from build123d import *

# Parameters (mm, degrees)
SKETCH2_W           = 75
SKETCH2_H           = 60
BOSS_EXTRUDE1_DEPTH = 2
SKETCH4_R           = 1.5
SKETCH4_R_2         = 2
CUT_EXTRUDE2_DEPTH  = 2
SKETCH5_R           = 5
CUT_EXTRUDE3_DEPTH  = 40
FILLET1_R           = 1


with BuildPart() as part:
    # Sketch2 → Boss-Extrude1 (new body)
    with BuildSketch(Plane(origin=(0, 0, 0), x_dir=(1, 0, 0), z_dir=(0, 1, 0))):
        with Locations((37.5, 30)):
            Rectangle(SKETCH2_W, SKETCH2_H)
    extrude(amount=BOSS_EXTRUDE1_DEPTH)

    # Sketch4 → Cut-Extrude2 (cut)
    with BuildSketch(Plane(origin=(0, 2, 0), x_dir=(1, 0, 0), z_dir=(0, 1, 0))):
        with Locations(Location((10, 10, 0), (0, 0, 270))):
            Circle(SKETCH4_R)
        with Locations(Location((65, 10, 0), (0, 0, 270))):
            Circle(SKETCH4_R)
        with Locations(Location((20, 20, 0), (0, 0, 270))):
            Circle(SKETCH4_R_2)
        with Locations(Location((55, 20, 0), (0, 0, 270))):
            Circle(SKETCH4_R_2)
        with Locations(Location((10, 50, 0), (0, 0, 270))):
            Circle(SKETCH4_R)
        with Locations(Location((65, 50, 0), (0, 0, 270))):
            Circle(SKETCH4_R)
    extrude(amount=-CUT_EXTRUDE2_DEPTH, mode=Mode.SUBTRACT)

    # Sketch5 → Cut-Extrude3 (cut)
    with BuildSketch(Plane(origin=(0, 2, 0), x_dir=(1, 0, 0), z_dir=(0, 1, 0))):
        with Locations(Location((37.5, 28, 0), (0, 0, 270))):
            Circle(SKETCH5_R)
    extrude(amount=-CUT_EXTRUDE3_DEPTH, mode=Mode.SUBTRACT)

    # Fillet1
    fillet1_edges = [part.edges().sort_by_distance(p)[0] for p in [
        (0, 1, -60),
        (75, 1, -60),
        (75, 1, 0),
        (0, 1, 0),
    ]]
    fillet(fillet1_edges, radius=FILLET1_R)


solid = part.part
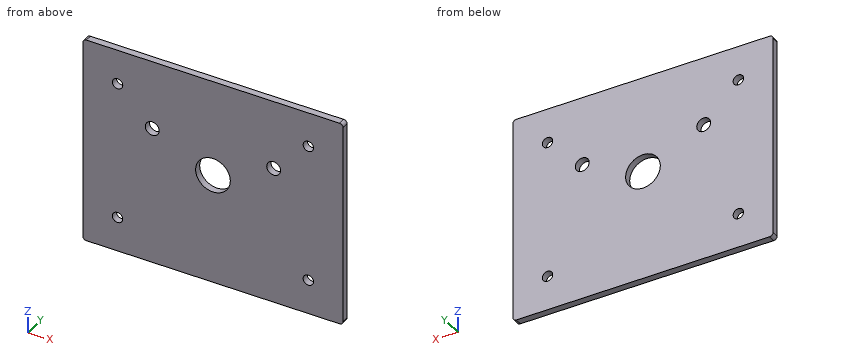
Source: CAD feature listing. Evaluate the final solid. Frame: model axes, mm. Round coordinates to 2 decimals unless told otherwise and drop trailing zeros. Loops run counter-clockwise (first coordinate to the right, second up) from the corner with the lowest first, then second, coordinate; pieces in that order, holes last.
Q1. Section D-D, the plane x = 55. Return loops of the section in (y, z), plus the area to 3 significant figures.
Q2. Ray query, line 1 (X direction, y = 1.4, z = -10); line 2 (X direction, y = 0.55, z = -20); line 3 (Z direction, x = 65, y = 0.9). Return the intervals inside material, ascending.
Q3. Section C-C, the plane y = 0.5. Return loops of the section in (x, z).
Q4. First-contact query: P1, Ø6.5, axis at x = 55, z = -20, coming from the +Y side. Flat tip, straight axial feed; report the tip coordinate or a pass-through.
Q5. Section B-B, the plane x = 65. Return loops of the section in (y, z), plus the area to 3 significant figures.
Q6. Section A-A, the plane z = -20. Return loops of the section in (x, y).
Solutions:
1. outline: (0, -60) - (2, -60) - (2, -22) - (0, -22) - close; (0, -18) - (2, -18) - (2, 0) - (0, 0) - close
1. area: 112 mm2
2. line 1: x = 0 to 8.5, 11.5 to 63.5, 66.5 to 75
2. line 2: x = 0 to 18, 22 to 53, 57 to 75
2. line 3: z = -60 to -51.5, -48.5 to -11.5, -8.5 to 0
3. outline: (0, -59) arc R1 ccw to (1, -60) - (74, -60) arc R1 ccw to (75, -59) - (75, -1) arc R1 ccw to (74, 0) - (1, 0) arc R1 ccw to (0, -1) - close; hole circle Ø3 at (10, -50); hole circle Ø3 at (10, -10); hole circle Ø4 at (20, -20); hole circle Ø10 at (37.5, -28); hole circle Ø4 at (55, -20); hole circle Ø3 at (65, -50); hole circle Ø3 at (65, -10)
4. P1: stops at y = 2
5. outline: (0, -60) - (2, -60) - (2, -51.5) - (0, -51.5) - close; (0, -48.5) - (2, -48.5) - (2, -11.5) - (0, -11.5) - close; (0, -8.5) - (2, -8.5) - (2, 0) - (0, 0) - close
5. area: 108 mm2
6. outline: (0, 0) - (18, 0) - (18, 2) - (0, 2) - close; (22, 0) - (53, 0) - (53, 2) - (22, 2) - close; (57, 0) - (75, 0) - (75, 2) - (57, 2) - close
